The listing builds one solid part. Answer for the finished solid, in the listing's coordinates (mm). Face numbers are marked on the shaded views. Round coordinates to 2 decimals unless told otherwise and drop trailing zeros. Loops run counter-clockwise (first coordinate to the right, second up) from the corner with the lowest first, then second, coordinate; pieces in that order, holes last. Notation, with made-up numbers: (50, -2) -> (59, -2) arc R36 ccw to (59, 36) -> close; hole circle Ø1 at (32.5, 70). An arc over 180 degrees is marked (long way). Use a Markdown table: item, result. Add a question column.
Q1. Section C-C on z = -63 is taken. Give the vertices of the cut face in (x, y), then the cut area to 3 significant figures.
Q2. Consider line 1 (Y direction, x = 0, z = -45); line 2 (X direction, y = -5, z = -56.5); line 3 (Y direction, x = 2, z = -30.5). Determine where each line is inside the solid, lowest interval first.
Q3. Given pin 1 Ø1 at (y, z) = (16, -87.5) entering from -X; pin 2 Ø1.5 at (x, z) = (-12, -54.5) entering from -Y; pin 3 Ø6 at (x, z) = (-14, -57.5) entering from -Y, each flat-ended and moving along its own axis, determine where each tip first touches the part or whether it passes through.
Q4. Section A-A on x = 0 is taken. Give the vertices of the cut face in (y, z).
Q5. For a pull along X with two mould halves and no side action, classify the marked faces 1, 2 and 3 as released by +X, released by -X, zero draft, split by the parting line, or undercut.
from build123d import *

# Parameters (mm, degrees)
EXTRUDE_1_DEPTH             = 5.5
SKETCH_2_R                  = 20
EXTRUDE_2_DEPTH             = 2
CHAMFER_1_SIZE              = 1.5
CHAMFER_1_SIZE2             = 1.787630389
CHAMFER_1_OF_MIRROR_1_SIZE2 = 1.5
CHAMFER_1_OF_MIRROR_1_SIZE  = 1.787630389
SKETCH_3_R                  = 3.4
CUT_EXTRUDE_1_DEPTH         = 30
SKETCH_8_R                  = 35
EXTRUDE_3_DEPTH             = 90
CUT_EXTRUDE_START           = -163
SKETCH_9_R                  = 3.4
CUT_EXTRUDE_2_DEPTH         = 163
FILLET_1_R                  = 2
SKETCH_10_R                 = 7.8
CUT_EXTRUDE_3_DEPTH         = 163
CHAMFER_2_SIZE              = 1
SKETCH_11_R                 = 106.702897297
CUT_EXTRUDE_4_DEPTH         = 322
CHAMFER_3_SIZE              = 1


with BuildPart() as part:
    # 스케치1 → 보스-돌출1 (new, symmetric)
    with BuildSketch(Plane.XY):
        with BuildLine():
            Line((12.279067203, 9.260056493), (13.72951471, 11.331510209))
            ThreePointArc((13.72951471, 11.331510209), (13.819231237, 11.644886966), (13.696740348, 11.946963163))
            ThreePointArc((13.696740348, 11.946963163), (12.880233507, 12.823034344), (12.007805037, 13.643432236))
            ThreePointArc((12.007805037, 13.643432236), (11.644638313, 13.792108644), (11.267252957, 13.684521298))
            Line((11.267252957, 13.684521298), (9.202645163, 12.238867358))
            ThreePointArc((9.202645163, 12.238867358), (8.915071795, 12.148443996), (8.627783828, 12.239770064))
            ThreePointArc((8.627783828, 12.239770064), (7.516754209, 12.951796446), (6.347354905, 13.563248531))
            ThreePointArc((6.347354905, 13.563248531), (6.081851507, 13.807041329), (6.003955886, 14.158977765))
            Line((6.003955886, 14.158977765), (6.224353416, 16.678133059))
            ThreePointArc((6.224353416, 16.678133059), (6.145361829, 16.994383555), (5.888243509, 17.194743772))
            ThreePointArc((5.888243509, 17.194743772), (4.743092252, 17.54519025), (3.577348088, 17.81946143))
            ThreePointArc((3.577348088, 17.81946143), (3.188498275, 17.766635614), (2.915466643, 17.484769561))
            Line((2.915466643, 17.484769561), (1.850290815, 15.200492627))
            ThreePointArc((1.850290815, 15.200492627), (1.646456756, 14.978397074), (1.351995179, 14.913843704))
            ThreePointArc((1.351995179, 14.913843704), (0.033801995, 14.974961851), (-1.284653671, 14.919795238))
            ThreePointArc((-1.284653671, 14.919795238), (-1.636482757, 14.998174295), (-1.879910562, 15.26401238))
            Line((-1.879910562, 15.26401238), (-2.948618349, 17.555863625))
            ThreePointArc((-2.948618349, 17.555863625), (-3.175152318, 17.790248795), (-3.498003423, 17.835206672))
            ThreePointArc((-3.498003423, 17.835206672), (-4.664956742, 17.566126596), (-5.811656393, 17.220780324))
            ThreePointArc((-5.811656393, 17.220780324), (-6.121997301, 16.980606919), (-6.217516604, 16.599987941))
            Line((-6.217516604, 16.599987941), (-5.997847464, 14.089158172))
            ThreePointArc((-5.997847464, 14.089158172), (-6.06332522, 13.794900649), (-6.286059898, 13.591765005))
            ThreePointArc((-6.286059898, 13.591765005), (-7.458207642, 12.985598321), (-8.572440333, 12.27859486))
            ThreePointArc((-8.572440333, 12.27859486), (-8.916322788, 12.170558572), (-9.260056493, 12.279067203))
            Line((-9.260056493, 12.279067203), (-11.331510209, 13.72951471))
            ThreePointArc((-11.331510209, 13.72951471), (-11.644886966, 13.819231237), (-11.946963163, 13.696740348))
            ThreePointArc((-11.946963163, 13.696740348), (-12.823034344, 12.880233507), (-13.643432236, 12.007805037))
            ThreePointArc((-13.643432236, 12.007805037), (-13.792108644, 11.644638313), (-13.684521298, 11.267252957))
            Line((-13.684521298, 11.267252957), (-12.238867358, 9.202645163))
            ThreePointArc((-12.238867358, 9.202645163), (-12.148443996, 8.915071795), (-12.239770064, 8.627783828))
            ThreePointArc((-12.239770064, 8.627783828), (-12.951796446, 7.516754209), (-13.563248531, 6.347354905))
            ThreePointArc((-13.563248531, 6.347354905), (-13.807041329, 6.081851507), (-14.158977765, 6.003955886))
            Line((-14.158977765, 6.003955886), (-16.678133059, 6.224353416))
            ThreePointArc((-16.678133059, 6.224353416), (-16.994383555, 6.145361829), (-17.194743772, 5.888243509))
            ThreePointArc((-17.194743772, 5.888243509), (-17.54519025, 4.743092252), (-17.81946143, 3.577348088))
            ThreePointArc((-17.81946143, 3.577348088), (-17.766635614, 3.188498275), (-17.484769561, 2.915466643))
            Line((-17.484769561, 2.915466643), (-15.200492627, 1.850290815))
            ThreePointArc((-15.200492627, 1.850290815), (-14.978397015, 1.646456653), (-14.913843726, 1.351994942))
            ThreePointArc((-14.913843726, 1.351994942), (-14.974961851, 0.033801876), (-14.919795238, -1.284653671))
            ThreePointArc((-14.919795238, -1.284653671), (-14.998174295, -1.636482757), (-15.26401238, -1.879910562))
            Line((-15.26401238, -1.879910562), (-17.555863625, -2.948618349))
            ThreePointArc((-17.555863625, -2.948618349), (-17.790248795, -3.175152318), (-17.835206672, -3.498003423))
            ThreePointArc((-17.835206672, -3.498003423), (-17.566126596, -4.664956742), (-17.220780324, -5.811656393))
            ThreePointArc((-17.220780324, -5.811656393), (-16.980606919, -6.121997301), (-16.599987941, -6.217516604))
            Line((-16.599987941, -6.217516604), (-14.089158172, -5.997847464))
            ThreePointArc((-14.089158172, -5.997847464), (-13.794900649, -6.06332522), (-13.591765005, -6.286059898))
            ThreePointArc((-13.591765005, -6.286059898), (-12.985598321, -7.458207642), (-12.27859486, -8.572440333))
            ThreePointArc((-12.27859486, -8.572440333), (-12.170558572, -8.916322788), (-12.279067203, -9.260056493))
            Line((-12.279067203, -9.260056493), (-13.72951471, -11.331510209))
            ThreePointArc((-13.72951471, -11.331510209), (-13.819231237, -11.644886966), (-13.696740348, -11.946963163))
            ThreePointArc((-13.696740348, -11.946963163), (-12.880233507, -12.823034344), (-12.007805037, -13.643432236))
            ThreePointArc((-12.007805037, -13.643432236), (-11.644638313, -13.792108644), (-11.267252957, -13.684521298))
            Line((-11.267252957, -13.684521298), (-9.202645163, -12.238867358))
            ThreePointArc((-9.202645163, -12.238867358), (-8.915071795, -12.148443996), (-8.627783828, -12.239770064))
            ThreePointArc((-8.627783828, -12.239770064), (-7.516754209, -12.951796446), (-6.347354905, -13.563248531))
            ThreePointArc((-6.347354905, -13.563248531), (-6.081851507, -13.807041329), (-6.003955886, -14.158977765))
            Line((-6.003955886, -14.158977765), (-6.224353416, -16.678133059))
            ThreePointArc((-6.224353416, -16.678133059), (-6.145361829, -16.994383555), (-5.888243509, -17.194743772))
            ThreePointArc((-5.888243509, -17.194743772), (-4.743092252, -17.54519025), (-3.577348088, -17.81946143))
            ThreePointArc((-3.577348088, -17.81946143), (-3.188498275, -17.766635614), (-2.915466643, -17.484769561))
            Line((-2.915466643, -17.484769561), (-1.850290815, -15.200492627))
            ThreePointArc((-1.850290815, -15.200492627), (-1.646456653, -14.978397015), (-1.351994942, -14.913843726))
            ThreePointArc((-1.351994942, -14.913843726), (-0.033801876, -14.974961851), (1.284653671, -14.919795238))
            ThreePointArc((1.284653671, -14.919795238), (1.636482757, -14.998174295), (1.879910562, -15.26401238))
            Line((1.879910562, -15.26401238), (2.948618349, -17.555863625))
            ThreePointArc((2.948618349, -17.555863625), (3.175152318, -17.790248795), (3.498003423, -17.835206672))
            ThreePointArc((3.498003423, -17.835206672), (4.664956742, -17.566126596), (5.811656393, -17.220780324))
            ThreePointArc((5.811656393, -17.220780324), (6.121997301, -16.980606919), (6.217516604, -16.599987941))
            Line((6.217516604, -16.599987941), (5.997847464, -14.089158172))
            ThreePointArc((5.997847464, -14.089158172), (6.06332522, -13.794900649), (6.286059898, -13.591765005))
            ThreePointArc((6.286059898, -13.591765005), (7.458207642, -12.985598321), (8.572440333, -12.27859486))
            ThreePointArc((8.572440333, -12.27859486), (8.916322788, -12.170558572), (9.260056493, -12.279067203))
            Line((9.260056493, -12.279067203), (11.331510209, -13.72951471))
            ThreePointArc((11.331510209, -13.72951471), (11.644886966, -13.819231237), (11.946963163, -13.696740348))
            ThreePointArc((11.946963163, -13.696740348), (12.823034344, -12.880233507), (13.643432236, -12.007805037))
            ThreePointArc((13.643432236, -12.007805037), (13.792108644, -11.644638313), (13.684521298, -11.267252957))
            Line((13.684521298, -11.267252957), (12.238867358, -9.202645163))
            ThreePointArc((12.238867358, -9.202645163), (12.148443996, -8.915071914), (12.239769926, -8.627784023))
            ThreePointArc((12.239769926, -8.627784023), (12.951796386, -7.516754312), (13.563248531, -6.347354905))
            ThreePointArc((13.563248531, -6.347354905), (13.807041329, -6.081851507), (14.158977765, -6.003955886))
            Line((14.158977765, -6.003955886), (16.678133059, -6.224353416))
            ThreePointArc((16.678133059, -6.224353416), (16.994383555, -6.145361829), (17.194743772, -5.888243509))
            ThreePointArc((17.194743772, -5.888243509), (17.54519025, -4.743092252), (17.81946143, -3.577348088))
            ThreePointArc((17.81946143, -3.577348088), (17.766635614, -3.188498275), (17.484769561, -2.915466643))
            Line((17.484769561, -2.915466643), (15.200492627, -1.850290815))
            ThreePointArc((15.200492627, -1.850290815), (14.978397015, -1.646456653), (14.913843726, -1.351994942))
            ThreePointArc((14.913843726, -1.351994942), (14.974961851, -0.033801876), (14.919795238, 1.284653671))
            ThreePointArc((14.919795238, 1.284653671), (14.998174295, 1.636482757), (15.26401238, 1.879910562))
            Line((15.26401238, 1.879910562), (17.555863625, 2.948618349))
            ThreePointArc((17.555863625, 2.948618349), (17.790248795, 3.175152318), (17.835206672, 3.498003423))
            ThreePointArc((17.835206672, 3.498003423), (17.566126596, 4.664956742), (17.220780324, 5.811656393))
            ThreePointArc((17.220780324, 5.811656393), (16.980606919, 6.121997301), (16.599987941, 6.217516604))
            Line((16.599987941, 6.217516604), (14.089158172, 5.997847464))
            ThreePointArc((14.089158172, 5.997847464), (13.794900649, 6.06332522), (13.591765005, 6.286059898))
            ThreePointArc((13.591765005, 6.286059898), (12.985598253, 7.458207762), (12.278594702, 8.572440559))
            ThreePointArc((12.278594702, 8.572440559), (12.170558572, 8.916322926), (12.279067203, 9.260056493))
        make_face()
    extrude(amount=EXTRUDE_1_DEPTH, both=True)

    # 스케치2 → 보스-돌출2 (add)
    with BuildSketch(Plane.XY.offset(5.5)):
        Circle(SKETCH_2_R)
    extrude_2 = extrude(amount=EXTRUDE_2_DEPTH)

    # 모따기1
    chamfer_1_edges = [part.edges().sort_by_distance(p)[0] for p in [
        (-20, 0, 5.5),
    ]]
    chamfer_1_side = [part.faces().sort_by_distance(p)[0] for p in [
        (-20, 0, 6.5),
    ]]
    chamfer(chamfer_1_edges, length=CHAMFER_1_SIZE, length2=CHAMFER_1_SIZE2, reference=chamfer_1_side[0])

    # 대칭 복사1: 보스-돌출2 across plane
    add(extrude_2.mirror(Plane.XY))

    # 모따기1 of 대칭 복사1
    chamfer_1_of_mirror_1_edges = [part.edges().sort_by_distance(p)[0] for p in [
        (-20, 0, -5.5),
    ]]
    chamfer(chamfer_1_of_mirror_1_edges, length=CHAMFER_1_OF_MIRROR_1_SIZE, length2=CHAMFER_1_OF_MIRROR_1_SIZE2)

    # 스케치3 → 컷-돌출1 (cut)
    with BuildSketch(Plane(origin=(0, 0, -7.5), x_dir=(-1, 0, 0), z_dir=(0, 0, -1))):
        Circle(SKETCH_3_R)
    extrude(amount=-CUT_EXTRUDE_1_DEPTH, mode=Mode.SUBTRACT)

    # 스케치8 → 보스-돌출3 (add)
    with BuildSketch(Plane(origin=(0, 0, -7.5), x_dir=(-1, 0, 0), z_dir=(0, 0, -1))):
        with Locations(Location((0, 0, 0), (0, 0, 180))):
            Circle(SKETCH_8_R)
    extrude(amount=EXTRUDE_3_DEPTH)

    # 스케치9 → 컷-돌출2 (cut)
    with BuildSketch(Plane.XY.offset(7.5).offset(CUT_EXTRUDE_START)):
        with Locations(Location((0, 0, 0), (0, 0, 180))):
            Circle(SKETCH_9_R)
    extrude(amount=CUT_EXTRUDE_2_DEPTH, mode=Mode.SUBTRACT)

    # 필렛1
    fillet_1_edges = [part.edges().sort_by_distance(p)[0] for p in [
        (-35, 0, -7.5),
        (-35, 0, -97.5),
    ]]
    fillet(fillet_1_edges, radius=FILLET_1_R)

    # 스케치10 → 컷-돌출3 (cut)
    with BuildSketch(Plane.XY.offset(7.5)):
        Circle(SKETCH_10_R)
    extrude(amount=-CUT_EXTRUDE_3_DEPTH, mode=Mode.SUBTRACT)

    # 모따기2
    chamfer_2_edges = [part.edges().sort_by_distance(p)[0] for p in [
        (-7.8, 0, 7.5),
        (-7.8, 0, -97.5),
    ]]
    chamfer(chamfer_2_edges, length=CHAMFER_2_SIZE)

    # 스케치11 → 컷-돌출4 (cut)
    with BuildSketch(Plane.XY.offset(-7.5)):
        Circle(SKETCH_11_R)
    extrude(amount=CUT_EXTRUDE_4_DEPTH, mode=Mode.SUBTRACT)

    # 모따기3
    chamfer_3_edges = [part.edges().sort_by_distance(p)[0] for p in [
        (-7.8, 0, -7.5),
    ]]
    chamfer(chamfer_3_edges, length=CHAMFER_3_SIZE)


solid = part.part
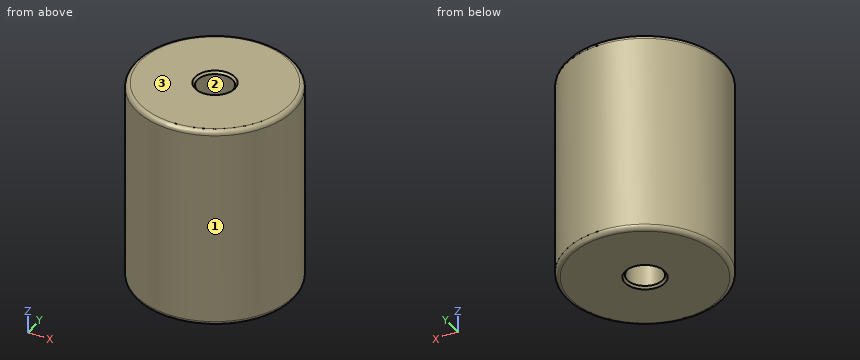
Checked values:
| question | item | result |
|---|---|---|
| 1 | outline | circle Ø70 at (0, 0); hole circle Ø15.6 at (0, 0) |
| 1 | area | 3,660 mm2 |
| 2 | line 1 | y = -35 to -7.8, 7.8 to 35 |
| 2 | line 2 | x = -34.64 to -5.99, 5.99 to 34.64 |
| 2 | line 3 | y = -34.94 to -7.54, 7.54 to 34.94 |
| 3 | pin 1 | stops at x = -31.38 |
| 3 | pin 2 | stops at y = -33.14 |
| 3 | pin 3 | stops at y = -33.23 |
| 4 | outline | (-35, -95.5) arc R2 ccw to (-33, -97.5) -> (-8.8, -97.5) -> (-7.8, -96.5) -> (-7.8, -8.5) -> (-8.8, -7.5) -> (-33, -7.5) arc R2 ccw to (-35, -9.5) -> close; (7.8, -96.5) -> (8.8, -97.5) -> (33, -97.5) arc R2 ccw to (35, -95.5) -> (35, -9.5) arc R2 ccw to (33, -7.5) -> (8.8, -7.5) -> (7.8, -8.5) -> close |
| 5 | face 1 | split by the parting line |
| 5 | face 2 | undercut |
| 5 | face 3 | zero draft |
